Here's how the part is built. I have some questions about the finished solid (model axes, mm). Round coordinates to 2 decimals unless told otherwise and drop trailing zeros. Write each loop counter-clockwise with the first axis right and the second up, starting at its lowest first coordinate (ties: lowest second). Pieces come first, ordered by that corner, then holes. Notation, with made-up numbers: (22.25, 35.25) - (63.25, 35.25) arc R19 ccw to (63.25, 51.25) - close; hole circle Ø10 at (51.5, 4.5). An arc over 180 degrees is marked (long way). One line per item, written item: value. Start each with the question number.
Item 1: Imagine slicing it at B-B, the plane z = 0. Please give me the cut outline in (x, y), then the cut area to 3 significant figures.
Item 2: If I drill on line 1 (Z direction, x = 16, y = 5.75); line 2 (X direction, y = 12.75, z = 1.25); line 3 (X direction, y = 1.75, z = -1), over which ranges is the centre line in solid material (lowest first)?
Item 3: Imagine slicing it at C-C, the plane x = -16. Please give me the cut outline in (y, z).
Item 4: Imagine slicing it at A-A, the plane y = 9. Please give me the cut outline in (x, z), then the cut area to 3 significant figures.
Item 5: Thinking about a two-plate mould opening in Z: for faces 1 (the face through (20, 10, 0)), 2 (the face through (-15.55, 9.86, 1.43)), 3 (the face through (0, 10, -6)), which applies, released by +Z, released by -Z, zero draft, split by the parting line, or undercut?
Item 6: For P1, Ø3.5, axis at x = 0, z = 0, coming from the -Y side, with a flat end and sliding along its axis, tell me the tip position at first contact or that it passes through.
Item 7: Imagine slicing it at D-D, the plane y = 3.25. Please give me the cut outline in (x, z).
```python
from build123d import *

# Parameters (mm, degrees)
SKETCH1_W           = 40
SKETCH1_H           = 12
SKETCH1_R           = 1.5
BOSS_EXTRUDE1_DEPTH = 20
SKETCH2_R           = 1.5
CUT_EXTRUDE1_DEPTH  = 20


with BuildPart() as part:
    # Sketch1 → Boss-Extrude1 (new body)
    with BuildSketch(Plane(origin=(0, 0, 0), x_dir=(1, 0, 0), z_dir=(0, 1, 0))):
        Rectangle(SKETCH1_W, SKETCH1_H)
        with Locations(Location((0, 0, 0), (0, 0, 270))):
            Circle(SKETCH1_R, mode=Mode.SUBTRACT)
        with Locations(Location((-16, 0, 0), (0, 0, 270))):
            Circle(SKETCH1_R, mode=Mode.SUBTRACT)
        with Locations(Location((16, 0, 0), (0, 0, 90))):
            Circle(SKETCH1_R, mode=Mode.SUBTRACT)
    extrude(amount=BOSS_EXTRUDE1_DEPTH)

    # Sketch2 → Cut-Extrude1 (cut)
    with BuildSketch(Plane(origin=(0, 0, -6), x_dir=(-1, 0, 0), z_dir=(0, 0, -1))):
        with Locations((10, 9)):
            Circle(SKETCH2_R)
        with Locations((-10, 9)):
            Circle(SKETCH2_R)
    extrude(amount=-CUT_EXTRUDE1_DEPTH, mode=Mode.SUBTRACT)


solid = part.part
```
Values follow:
1. outline: (-20, 0) - (-17.5, 0) - (-17.5, 20) - (-20, 20) - close; (-14.5, 0) - (-1.5, 0) - (-1.5, 20) - (-14.5, 20) - close; (1.5, 0) - (14.5, 0) - (14.5, 20) - (1.5, 20) - close; (17.5, 0) - (20, 0) - (20, 20) - (17.5, 20) - close; hole circle Ø3 at (-10, 9); hole circle Ø3 at (10, 9)
1. area: 606 mm^2
2. line 1: z = -6 to -1.5, 1.5 to 6
2. line 2: x = -20 to -16.83, -15.17 to -0.83, 0.83 to 15.17, 16.83 to 20
2. line 3: x = -20 to -17.12, -14.88 to -1.12, 1.12 to 14.88, 17.12 to 20
3. outline: (0, -6) - (20, -6) - (20, -1.5) - (0, -1.5) - close; (0, 1.5) - (20, 1.5) - (20, 6) - (0, 6) - close
4. outline: (-20, -6) - (-11.5, -6) - (-11.5, 6) - (-20, 6) - close; (-8.5, -6) - (8.5, -6) - (8.5, 6) - (-8.5, 6) - close; (11.5, -6) - (20, -6) - (20, 6) - (11.5, 6) - close; hole circle Ø3 at (-16, 0); hole circle Ø3 at (0, 0); hole circle Ø3 at (16, 0)
4. area: 387 mm^2
5. face 1: zero draft
5. face 2: undercut
5. face 3: released by -Z
6. P1: stops at y = 0
7. outline: (-20, -6) - (20, -6) - (20, 6) - (-20, 6) - close; hole circle Ø3 at (-16, 0); hole circle Ø3 at (0, 0); hole circle Ø3 at (16, 0)
